```python
from build123d import *

# Parameters (mm, degrees)
F0_R     = 115
F1_DEPTH = 70
F2_R     = 17.5
F3_DEPTH = 7
F5_R     = 10
F6_R     = 115
F6_R_2   = 110
F7_DEPTH = 10


# Not quite as in the source:
# - a fillet or chamfer that OpenCascade refuses, or shapes differently, is made with other operations: its cross-section is extruded or revolved along the edge and cut away or added


with BuildPart() as f1:
    # F0 (on Top) → F1 (new body)
    with BuildSketch(Plane.XY):
        Circle(F0_R)
    extrude(amount=F1_DEPTH)

    # F2 (on face) → F3 (cut)
    with BuildSketch(Plane(origin=(0, 0, 0), x_dir=(1, 0, 0), z_dir=(0, 0, -1))):
        with Locations((-60, 60)):
            Circle(F2_R)
        with Locations((-60, -60)):
            Circle(F2_R)
        with Locations((60, -60)):
            Circle(F2_R)
        with Locations((60, 60)):
            Circle(F2_R)
    extrude(amount=-F3_DEPTH, mode=Mode.SUBTRACT)

    # F4: fillet of radius 12 on 4 edges, made by hand

    # F4_s1 → F4_t2 (revolve)
    with BuildSketch(Plane.XZ.offset(60)):
        with BuildLine():
            ThreePointArc((-42.5, 0), (-46.9279714162, 5.0995049384), (-53.4087121146, 7))
            Line((-53.4087121146, 7), (-42.5, 7))
            Line((-42.5, 7), (-42.5, 0))
        make_face()
    revolve(axis=Axis((-60, -60, 7), (0, 0, -1)))

    # F4_s3 → F4_t4 (revolve)
    with BuildSketch(Plane.XZ.offset(-60)):
        with BuildLine():
            ThreePointArc((-42.5, 0), (-46.9279714162, 5.0995049384), (-53.4087121146, 7))
            Line((-53.4087121146, 7), (-42.5, 7))
            Line((-42.5, 7), (-42.5, 0))
        make_face()
    revolve(axis=Axis((-60, 60, 7), (0, 0, -1)))

    # F4_s5 → F4_t6 (revolve)
    with BuildSketch(Plane.XZ.offset(-60)):
        with BuildLine():
            ThreePointArc((77.5, 0), (73.0720285838, 5.0995049384), (66.5912878854, 7))
            Line((66.5912878854, 7), (77.5, 7))
            Line((77.5, 7), (77.5, 0))
        make_face()
    revolve(axis=Axis((60, 60, 7), (0, 0, -1)))

    # F4_s7 → F4_t8 (revolve)
    with BuildSketch(Plane.XZ.offset(60)):
        with BuildLine():
            ThreePointArc((77.5, 0), (73.0720285838, 5.0995049384), (66.5912878854, 7))
            Line((66.5912878854, 7), (77.5, 7))
            Line((77.5, 7), (77.5, 0))
        make_face()
    revolve(axis=Axis((60, -60, 7), (0, 0, -1)))

    # F5
    f5_edges = [f1.edges().sort_by_distance(p)[0] for p in [
        (-115, 0, 70),
    ]]
    fillet(f5_edges, radius=F5_R)

    # F6 (on face) → F7 (cut)
    with BuildSketch(Plane(origin=(0, 0, 0), x_dir=(1, 0, 0), z_dir=(0, 0, -1))):
        Circle(F6_R)
        Circle(F6_R_2, mode=Mode.SUBTRACT)
    extrude(amount=-F7_DEPTH, mode=Mode.SUBTRACT)


solid = f1.part
```
Can you work these out from the model? Positions are in its coordinate system, mm. A direction names the side the tool comes from. Coordinates: 2 decimals unless noted, no trailing zeros. Loops run counter-clockwise (first coordinate to the right, second up) from the corner with the lowest first, then second, coordinate; pieces in that order, holes last. Notation, with made-up numbers: (63.5, 78) -> (109.5, 78) arc R20 ccw to (109.5, 116) -> close; hole circle Ø9 at (49.5, -2). An arc over 180 degrees is marked (long way). Answer as a JSON object with one key per item and string values.
1) For faces 1 (the face through (-2, 2, 0)), 2 (the face through (60, 60, 7)), which set-ups out of +Z, -Z, +X, -X, +Y, -Y let a thin tool reach every point of the face, with its end or its side?
Results:
{"face 1": "-Z, +X, -X, +Y, -Y", "face 2": "-Z"}
2) Imagine slicing it at A-A (z = 34.5). Please give me the cut outline in (x, y), then the cut area to 3 significant figures.
Results:
{"outline": "circle Ø230 at (0, 0)", "area": "41,500 mm^2"}
3) Thinking about a two-plate mould opening in X: for faces 3 (the face through (60, -60, 7)), 4 (the face through (-60, -60, 7)), 5 (the face through (-24.93, -112.265, 34.65)), 6 (the face through (-1, 1, 70)), which applies, pulls with the +X half, pulls with the -X half, needs draft (parallel to the pull), parting line crosses it, or undercut?
Results:
{"face 3": "undercut", "face 4": "undercut", "face 5": "parting line crosses it", "face 6": "needs draft"}
4) If I drill on line 1 (Y direction, x = -47, z = 23); line 2 (Z direction, x = 51, y = 47); line 3 (Y direction, x = 27.5, z = 13), over which ranges is the centre line in solid material (lowest first)?
Results:
{"line 1": "y = -104.96 to 104.96", "line 2": "z = 2.68 to 70", "line 3": "y = -111.66 to 111.66"}
5) For P1, Ø10.5, axis at x = -62.5, y = -63, coming from the -Z side; P2, Ø10.5, axis at x = 58.5, y = 59, coming from the -Z side; P3, Ø1, axis at x = 61, y = -86.5, coming from the +Z side; P4, Ø10, axis at x = 58, y = 84.5, coming from the -Z side, each with a flat end and sliding along its axis, tell me the tip position at first contact or that it passes through.
Results:
{"P1": "stops at z = 6.72", "P2": "stops at z = 6.99", "P3": "stops at z = 69.99", "P4": "stops at z = 0"}
